Could you check a few things on this drawing? It's one solid part, dimensions in mm from its lowest x, y, z. A direction names the side the tool comes from. Coordinates: 2 decimals unless noted, no trailing zeros. Loops run counter-clockwise (first coordinate to the right, second up) from the corner with the lowest first, then second, coordinate; pieces in that order, holes last. Notation, with made-up numbers: (-16, 76.5) -> (35, 76.5) arc R18 cw to (35, 93.5) -> close; hole circle Ø10 at (51.5, 54). An arc over 180 degrees is marked (long way). One line per question, with ' | ' between items. Start each with the question number.
(1) Suppose I cut it at C-C (x = 6). Please give me the cut outline in (y, z) (1 decimal).
(2) If I drill on line 1 along Y through (x, z) = (20, 9.75); line 2 along Y through (x, z) = (12, 19); line 3 along Z through (x, y) = (18.5, 28.5), over which ranges is the centre line in solid material (lowest first)?
(3) If we mould it in two halves opening along X, with no side actions, what happens to the marked faces 1, 2 and 3? For each: pulls with the +X half, pulls with the -X half, needs draft (parallel to the pull), parting line crosses it, or undercut.
(4) Suppose I cut it at A-A (x = 20). Please give me the cut outline in (y, z), plus the area to 3 significant figures.
(5) Which directions (+Z, -Z, +X, -X, +Y, -Y) give clear straight access to the entire face, cutting with the end or side of a thin tool? Please do the marked faces 4 and 5.
(6) I'm going to push flat-ended pins straight in: pin 1 Ø0.9 at (x, y) = (3.5, 12) entering from +Z; pin 2 Ø1.5 at (y, z) = (5.5, 13.5) entering from +X (1 decimal); pin 3 Ø8 at (x, z) = (17, 18) entering from +Y; pin 4 Ø7.5 at (x, y) = (20, 20) entering from -Z. Where does each tip first touch, or does it pass through?
(7) Suppose I cut it at D-D (z = 4). Please give me the cut outline in (x, y), plus the area to 3 significant figures.
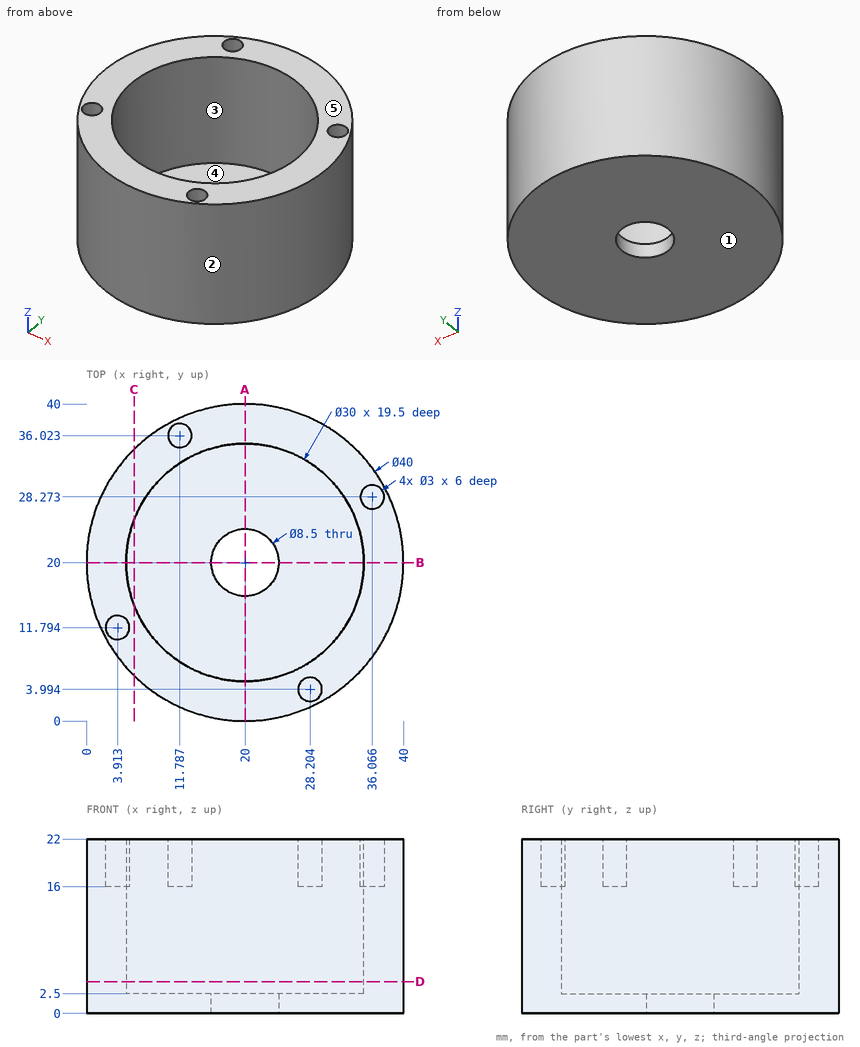
Checks:
1) outline: (5.7, 0) -> (34.3, 0) -> (34.3, 22) -> (25.4, 22) -> (25.4, 2.5) -> (14.6, 2.5) -> (14.6, 22) -> (5.7, 22) -> close
2) line 1: y = 0 to 5, 35 to 40 | line 2: y = 1.67 to 7.31, 32.69 to 34.54, 37.51 to 38.33 | line 3: z = 0 to 2.5
3) face 1: needs draft | face 2: parting line crosses it | face 3: undercut
4) outline: (0, 0) -> (15.75, 0) -> (15.75, 2.5) -> (5, 2.5) -> (5, 22) -> (0, 22) -> close; (24.25, 0) -> (40, 0) -> (40, 22) -> (35, 22) -> (35, 2.5) -> (24.25, 2.5) -> close | area: 274 mm^2
5) face 4: +Z | face 5: +Z, +X, -X, +Y, -Y
6) pin 1: stops at z = 16 | pin 2: stops at x = 34.5 | pin 3: stops at y = 40 | pin 4: passes through
7) outline: circle Ø40 at (20, 20); hole circle Ø30 at (20, 20) | area: 550 mm^2
